```python
from build123d import *

# Parameters (mm, degrees)
SKETCH1_W                  = 229
SKETCH1_H                  = 120
BOSS_EXTRUDE1_DEPTH        = 5
SKETCH4_W                  = 20.632503002
SKETCH4_H                  = 53.730004003
BOSS_EXTRUDE2_DEPTH        = 10
F_16_0_16_DIAMETER_HOLE1_D = 16
M6_CLEARANCE_HOLE1_D       = 6.4


with BuildPart() as part:
    # Sketch1 → Boss-Extrude1 (new, symmetric)
    with BuildSketch(Plane(origin=(0, 0, 0), x_dir=(1, 0, 0), z_dir=(0, 1, 0))):
        with Locations((-114.5, 0)):
            Rectangle(SKETCH1_W, SKETCH1_H)
    extrude(amount=BOSS_EXTRUDE1_DEPTH, both=True)

    # Sketch4 → Boss-Extrude2 (add)
    with BuildSketch(Plane(origin=(0, 5, 0), x_dir=(1, 0, 0), z_dir=(0, 1, 0))):
        with Locations((10.316251501, 33.134997999)):
            Rectangle(SKETCH4_W, SKETCH4_H)
    extrude(amount=-BOSS_EXTRUDE2_DEPTH)

    # Ø16.0 (16) Diameter Hole1 (through all)
    with Locations(Plane(origin=(0, 5, 0), x_dir=(1, 0, 0), z_dir=(0, 1, 0))):
        with Locations((-213, 44), (-147.323, 44), (-81.646, 44), (-15.969, 44), (-213, -44), (-147.323, -44), (-81.646, -44), (-15.969, -44)):
            Hole(F_16_0_16_DIAMETER_HOLE1_D / 2)

    # M6 Clearance Hole1 (through all)
    with Locations(Plane(origin=(0, 5, 0), x_dir=(1, 0, 0), z_dir=(0, 1, 0))):
        with Locations((-199.875, 16.78), (-157.875, 16.78), (-119.875, 9.852366083), (-77.875, 9.852366083), (-39.875, 20.69101), (2.125, 20.69101)):
            Hole(M6_CLEARANCE_HOLE1_D / 2)


solid = part.part
```
Geometry check sheet. Reference: the model listing, model coordinates, mm. A direction names the side the tool comes from. Give positions to 0.01 mm unless a question says otherwise; leave off trailing zeros. Order: outer loops, then holes, each group sorted by start corner. A loop starts at its lowest first (then second) coordinate and runs counter-clockwise, first axis right, second up.
1. Thickness scan on L1, parallel to X at y = -3, z = 44; L2, parallel to Z at x = -213, y = 2.25; L3, parallel to Z at x = -12.5, y = 2. Record the ranges inside material, lowest first.
2. Section check C-C, the plane y = -0.25. Give the number of separate pieces and of enclosed holes in the cut face, and give its area (3 significant figures).
3. Section check A-A, the plane x = -213. Enter the section's corners in (y, z).
4. Release check for a two-part mould opening along Z. For faces 3 (the face through (-229, 0, 1)), 4 (the face through (-77.458, -0.07, -13.025)), 5 (the face through (-116, 0, 60)), 6 (the face through (-211.959, -0.07, -51.932)) record: pulls with the +Z half, pulls with the -Z half, needs draft (parallel to the pull), parting line crosses it, or undercut.
5. Gauge pin test, flat end, axial feed: pin 1 Ø3 at (x, y) = (6, -0.5) entering from +Z. Record the tip position at first contact, or that the pin passes through.
6. Section check D-D, the plane z = 25. Enter the section's corners in (x, y), and give its area (3 significant figures).
7. Section check B-B, the plane z = -38.5. Enter the section's corners in (x, y).
8. Access from +Z, -Z, +X, -X, +Y, -Y to the whole of each face (thin tool, end or side, straight path). Record for faces 1 (the face through (-106, 5, -1)), 2 (the face through (10, 0, -6.27)).
Values follow:
1. L1: x = -229 to -221, -205 to -155.32, -139.32 to -89.65, -73.65 to -23.97, -7.97 to 0
1. L2: z = -60 to -52, -36 to 36, 52 to 60
1. L3: z = -60 to -51.21, -36.79 to 36.79, 51.21 to 60
2. separate pieces: 1
2. enclosed holes: 14
2. area: 26,800 mm2
3. outline: (-5, -60) - (5, -60) - (5, -52) - (-5, -52) - close; (-5, -36) - (5, -36) - (5, 36) - (-5, 36) - close; (-5, 52) - (5, 52) - (5, 60) - (-5, 60) - close
4. face 3: needs draft
4. face 4: undercut
4. face 5: pulls with the +Z half
4. face 6: undercut
5. pin 1: stops at z = -6.27
6. outline: (-229, -5) - (0, -5) - (0, 5) - (-229, 5) - close
6. area: 2,290 mm2
7. outline: (-229, -5) - (-218.81, -5) - (-218.81, 5) - (-229, 5) - close; (-207.19, -5) - (-153.13, -5) - (-153.13, 5) - (-207.19, 5) - close; (-141.51, -5) - (-87.46, -5) - (-87.46, 5) - (-141.51, 5) - close; (-75.84, -5) - (-21.78, -5) - (-21.78, 5) - (-75.84, 5) - close; (-10.16, -5) - (20.63, -5) - (20.63, 5) - (-10.16, 5) - close
8. face 1: +Z, -Z, +X, -X, +Y
8. face 2: +Z, +X, +Y, -Y
